Geometry: final body of the model. Coordinates: model frame, mm. Face numbers are marked on the shaded views. A direction names the side the tool comes from. Give positions to 0.01 mm unless a question says otherwise; leave off trailing zeros. Order: outer loops, then holes, each group sorted by start corner. A loop starts at its lowest first (then second) coordinate and runs counter-clockwise, first axis right, second up. Notation, with made-up numbers: (10.25, -17.75) - (20.25, -17.75) arc R30 ccw to (20.25, 10.25) - close; hole circle Ø8 at (-16, 80.25). An arc over 180 degrees is marked (long way). One line per question, with ' | ' between items. Start each with the question number.
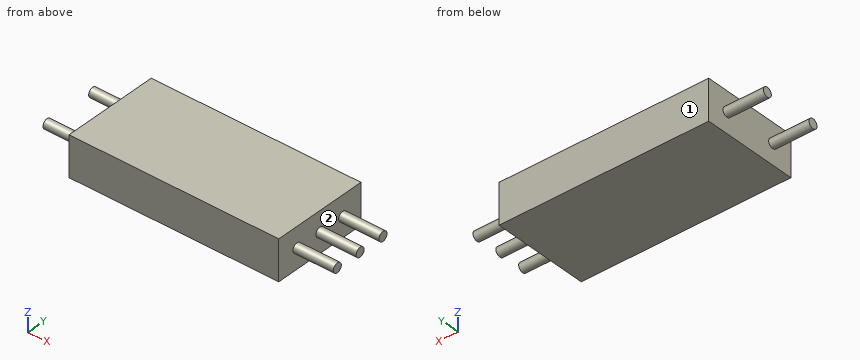
from build123d import *

# Parameters (mm, degrees)
SKETCH_2_W      = 78
SKETCH_2_H      = 36
EXTRUDE_1_DEPTH = 7.5
SKETCH_3_R      = 1.75
EXTRUDE_2_DEPTH = 15
EXTRUDE_START   = 15
SKETCH_4_R      = 1.75
EXTRUDE_3_DEPTH = 15


with BuildPart() as part:
    # Эскиз2 → Бобышка-Вытянуть1 (new, symmetric)
    with BuildSketch(Plane.XY):
        Rectangle(SKETCH_2_W, SKETCH_2_H)
    extrude(amount=EXTRUDE_1_DEPTH, both=True)

    # Эскиз3 → Бобышка-Вытянуть2 (add)
    with BuildSketch(Plane(origin=(39, 0, 0), x_dir=(0, 0, -1), z_dir=(1, 0, 0))):
        with Locations(Location((0, -10, 0), (0, 0, 180))):
            Circle(SKETCH_3_R)
        with Locations(Location((0, 0, 0), (0, 0, 180))):
            Circle(SKETCH_3_R)
        with Locations(Location((0, 10, 0), (0, 0, 180))):
            Circle(SKETCH_3_R)
    extrude(amount=EXTRUDE_2_DEPTH)

    # Эскиз4 → Бобышка-Вытянуть3 (add)
    with BuildSketch(Plane.ZY.offset(39).offset(EXTRUDE_START)):
        with Locations((0, 10)):
            Circle(SKETCH_4_R)
        with Locations((0, -10)):
            Circle(SKETCH_4_R)
    extrude(amount=-EXTRUDE_3_DEPTH)


solid = part.part
(1) Material intervals for line 1 along X through (y, z) = (-9.5, 4.25), sorted ascending. Write a range as from..to.
(2) Cut plane A-A, the plane y = 0. Return the cut outline in (x, z), plus the area to 3 significant figures.
(3) Cut plane C-C, the plane y = 10. Return the cut outline in (x, z).
(4) Access query for the marked faces 1 and 2. Directions: +Z, -Z, +X, -X, +Y, -Y. A direction counts if a zero-diameter tool reaches every point of the face in a straight line with its end or side. Return the directions, or none.
(5) Cut plane B-B, the plane z = 0. Return the cut outline in (x, y).
(6) Cut plane D-D, the plane y = -5.5. Return the cut outline in (x, z), plus the area to 3 significant figures.
Results are:
1) line 1: -39..39
2) outline: (-39, -7.5) - (39, -7.5) - (39, -1.75) - (54, -1.75) - (54, 1.75) - (39, 1.75) - (39, 7.5) - (-39, 7.5) - close | area: 1,220 mm2
3) outline: (-54, -1.75) - (-39, -1.75) - (-39, -7.5) - (39, -7.5) - (39, -1.75) - (54, -1.75) - (54, 1.75) - (39, 1.75) - (39, 7.5) - (-39, 7.5) - (-39, 1.75) - (-54, 1.75) - close
4) face 1: +Z, -Z, +X, -X, +Y | face 2: +X
5) outline: (-54, -11.75) - (-39, -11.75) - (-39, -18) - (39, -18) - (39, -11.75) - (54, -11.75) - (54, -8.25) - (39, -8.25) - (39, -1.75) - (54, -1.75) - (54, 1.75) - (39, 1.75) - (39, 8.25) - (54, 8.25) - (54, 11.75) - (39, 11.75) - (39, 18) - (-39, 18) - (-39, 11.75) - (-54, 11.75) - (-54, 8.25) - (-39, 8.25) - (-39, -8.25) - (-54, -8.25) - close
6) outline: (-39, -7.5) - (39, -7.5) - (39, 7.5) - (-39, 7.5) - close | area: 1,170 mm2
